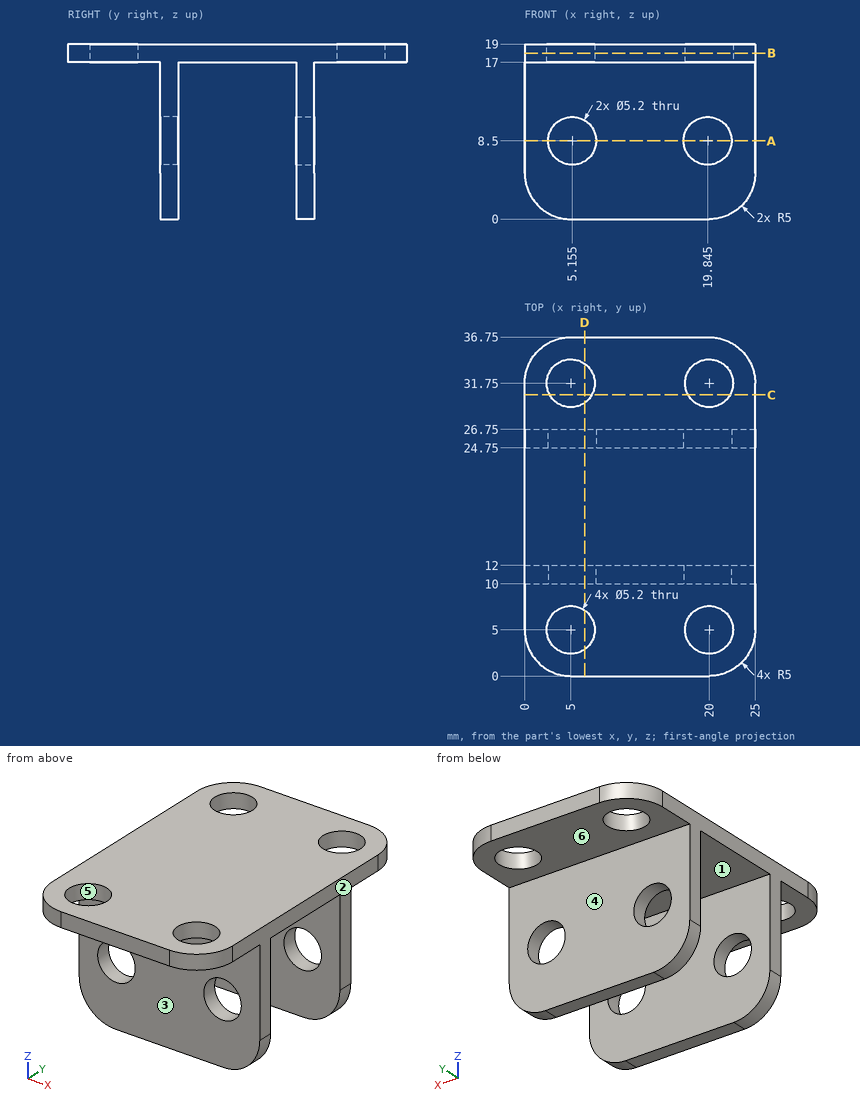
Geometry: see drawing. Coordinates: mm, zero at the bounding-box minimum. A direction names the side the tool comes from. Give positions to 0.01 mm unless a question says otherwise; leave off trailing zeros. Order: outer loops, then holes, each group sorted by start corner. A loop starts at its lowest first (then second) coordinate and runs counter-clockwise, first axis right, second up. Notation, with made-up numbers: M 87,80.25 L 91,80.25 A22 cw 91,95.25 Z; hole C 2,38 d6. An arc over 180 degrees is marked long. Answer as a JSON object with one key per item and string values.
1. Cut plane C-C, the plane y = 30.5. Output: boundary loops of the cut face in (x, z).
Result sheet:
{"outline": "M 0,17 L 2.72,17 L 2.72,19 L 0,19 Z; M 7.28,17 L 17.72,17 L 17.72,19 L 7.28,19 Z; M 22.28,17 L 25,17 L 25,19 L 22.28,19 Z"}
2. Reachability of the marked faces 1, 2 and 3 from +Z, -Z, +X, -X, +Y, -Y: full face, straight path, thin tool, end or side. Return the list, or none.
Result sheet:
{"face 1": "-Z, +X, -X", "face 2": "+Z, -Z, +X, +Y, -Y", "face 3": "-Z, +X, -X, -Y"}
3. Pull-direction query (Y, two-part tool) for the marked faces 4, 5 and 6; classes: +Y half, -Y half, draft (parallel to the pull), parting line (faces both ways), or undercut.
Result sheet:
{"face 4": "+Y half", "face 5": "undercut", "face 6": "draft"}
4. Cut plane D-D, the plane x = 6.5. Output: boundary loops of the cut face in (y, z), and give its area (3 significant figures).
Result sheet:
{"outline": "M 0,17 L 2.88,17 L 2.88,19 L 0,19 Z; M 7.12,17 L 10,17 L 10,10.73 L 12,10.73 L 12,17 L 24.75,17 L 24.75,10.73 L 26.75,10.73 L 26.75,17 L 29.63,17 L 29.63,19 L 7.12,19 Z; M 10,0 L 12,0 L 12,6.27 L 10,6.27 Z; M 24.75,0 L 26.75,0 L 26.75,6.27 L 24.75,6.27 Z; M 33.87,17 L 36.75,17 L 36.75,19 L 33.87,19 Z", "area": "107 mm²"}
5. Cut plane B-B, the plane z = 18. Output: boundary loops of the cut face in (x, y), and give its area (3 significant figures).
Result sheet:
{"outline": "M 0,5 A5 ccw 5,0 L 20,0 A5 ccw 25,5 L 25,31.75 A5 ccw 20,36.75 L 5,36.75 A5 ccw 0,31.75 Z; hole C 5,5 d5.2; hole C 5,31.75 d5.2; hole C 20,5 d5.2; hole C 20,31.75 d5.2", "area": "812 mm²"}
6. Cut plane A-A, the plane z = 8.5. Output: boundary loops of the cut face in (x, y) (3 decimals).
Result sheet:
{"outline": "M 0,10 L 2.555,10 L 2.555,12 L 0,12 Z; M 0,24.75 L 2.555,24.75 L 2.555,26.75 L 0,26.75 Z; M 7.755,10 L 17.245,10 L 17.245,12 L 7.755,12 Z; M 7.755,24.75 L 17.245,24.75 L 17.245,26.75 L 7.755,26.75 Z; M 22.445,10 L 25,10 L 25,12 L 22.445,12 Z; M 22.445,24.75 L 25,24.75 L 25,26.75 L 22.445,26.75 Z"}
7. Ray query, line 1 (Y direction, x = 20, z = 17.65); line 2 (X direction, y = 11.3, z = 8.5) (3 decimals). Return the intervals inside material, ascending. Write a range as [from, to].
Result sheet:
{"line 1": "[0, 2.4], [7.6, 29.15], [34.35, 36.75]", "line 2": "[0, 2.555], [7.755, 17.245], [22.445, 25]"}
8. First-contact query: P1, Ø4, axis at x = 11, y = 15.5, coming from the -Z side; P2, Ø10, axis at y = 28.5, z = 11, coming from the -X side; P3, Ø3, axis at x = 5, y = 31.75, coming from the +Z side; P4, Ø8.5, axis at x = 19.845, z = 8.5, coming from the -Y side. Flat tips, straight axial feed; report the tip coordinate or a pass-through.
Result sheet:
{"P1": "z = 17", "P2": "x = 0", "P3": "through", "P4": "y = 10"}
